Read the model definition and answer for the solid it produces. Units are mm, in the model's axes. Give positions to 0.01 mm unless a question says otherwise; leave off trailing zeros. Order: outer loops, then holes, each group sorted by start corner. A loop starts at its lowest first (then second) coordinate and runs counter-clockwise, first axis right, second up. Notation, with made-up numbers: (46.25, 41) - (77.25, 41) arc R31 ccw to (77.25, 70) - close; hole circle Ø9 at (77.5, 19). An arc over 180 degrees is marked (long way). Use a Markdown table: item, result. Add a question column.
1. A cutting plane is placed at B-B on x = 126.5. Determine the outline of the cut face in (y, z), and give its area (3 significant figures).
2. A flat-ended cylindrical pin translates along its axis: P1, Ø6, axis at x = 304.5, z = 17.5, coming from the +Y side. Find the tip coordinate at first contact, or state that the pin passes through.
3. A cutting plane is placed at A-A on z = 108.5. Determine the outline of the cut face in (x, y), and give its area (3 significant figures).
4. A cutting plane is placed at D-D on y = 2.55. State how many separate pieces and enclosed holes the cut face has, and give its area (3 significant figures).
5. Consider L1, parallel to Z at x = 110.5, y = 1; L2, parallel to X at y = 0.9, z = 93; L3, parallel to Z at x = 262, y = 2.75. Determine where each line is inside the solid, lowest interval first.
6. A cutting plane is placed at C-C on x = 291. Determine the outline of the cut face in (y, z), and give its area (3 significant figures).
```python
from build123d import *

# Parameters (mm, degrees)
SKETCH1_W           = 334.17
SKETCH1_H           = 162.4
BOSS_EXTRUDE1_DEPTH = 3
SKETCH2_R           = 5
CUT_EXTRUDE1_DEPTH  = 17
SKETCH3_W           = 3
SKETCH3_H           = 9.7
CUT_EXTRUDE3_DEPTH  = 45


with BuildPart() as part:
    # Sketch1 → Boss-Extrude1 (new body)
    with BuildSketch(Plane(origin=(0, 0, 0), x_dir=(1, 0, 0), z_dir=(0, 1, 0))):
        with Locations((167.085, -81.2)):
            Rectangle(SKETCH1_W, SKETCH1_H)
    extrude(amount=BOSS_EXTRUDE1_DEPTH)

    # Sketch2 → Cut-Extrude1 (cut)
    with BuildSketch(Plane(origin=(0, 0, 0), x_dir=(1, 0, 0), z_dir=(0, 1, 0))):
        with Locations((210, -17.5)):
            Circle(SKETCH2_R)
        with Locations((223.5, -17.5)):
            Circle(SKETCH2_R)
        with Locations((237, -17.5)):
            Circle(SKETCH2_R)
        with Locations((250.5, -17.5)):
            Circle(SKETCH2_R)
        with Locations((264, -17.5)):
            Circle(SKETCH2_R)
        with Locations((277.5, -17.5)):
            Circle(SKETCH2_R)
        with Locations((291, -17.5)):
            Circle(SKETCH2_R)
        with Locations((304.5, -17.5)):
            Circle(SKETCH2_R)
        with Locations((223.5, -35)):
            Circle(SKETCH2_R)
        with Locations((237, -35)):
            Circle(SKETCH2_R)
        with Locations((250.5, -35)):
            Circle(SKETCH2_R)
        with Locations((264, -35)):
            Circle(SKETCH2_R)
        with Locations((277.5, -35)):
            Circle(SKETCH2_R)
        with Locations((291, -35)):
            Circle(SKETCH2_R)
        with Locations((304.5, -35)):
            Circle(SKETCH2_R)
        with Locations((210, -35)):
            Circle(SKETCH2_R)
        with Locations((318, -17.5)):
            Circle(SKETCH2_R)
        with Locations((318, -35)):
            Circle(SKETCH2_R)
        with BuildLine():
            Line((210, -47.5), (255, -47.5))
            ThreePointArc((255, -47.5), (260, -52.5), (255, -57.5))
            Line((255, -57.5), (210, -57.5))
            ThreePointArc((210, -57.5), (205, -52.5), (210, -47.5))
        make_face()
        with BuildLine():
            Line((275, -57.5), (320, -57.5))
            ThreePointArc((320, -57.5), (325, -52.5), (320, -47.5))
            Line((320, -47.5), (275, -47.5))
            ThreePointArc((275, -47.5), (270, -52.5), (275, -57.5))
        make_face()
        with BuildLine():
            Line((15, -17.2), (60, -17.2))
            ThreePointArc((60, -17.2), (65, -12.2), (60, -7.2))
            Line((60, -7.2), (15, -7.2))
            ThreePointArc((15, -7.2), (10, -12.2), (15, -17.2))
        make_face()
        with BuildLine():
            Line((95, -7.2), (140, -7.2))
            ThreePointArc((140, -7.2), (145, -12.2), (140, -17.2))
            Line((140, -17.2), (95, -17.2))
            ThreePointArc((95, -17.2), (90, -12.2), (95, -7.2))
        make_face()
    cut_extrude1 = extrude(amount=CUT_EXTRUDE1_DEPTH, mode=Mode.SUBTRACT)

    # Mirror1: Cut-Extrude1 across plane
    add(cut_extrude1.mirror(Plane.XY.offset(81.2)), mode=Mode.SUBTRACT)

    # Sketch3 → Cut-Extrude3 (cut)
    with BuildSketch(Plane(origin=(0, 0, 0), x_dir=(1, 0, 0), z_dir=(0, 1, 0))):
        with Locations((204.7, -69.2)):
            Rectangle(SKETCH3_W, SKETCH3_H)
        with Locations((204.7, -93.2)):
            Rectangle(SKETCH3_W, SKETCH3_H)
    extrude(amount=CUT_EXTRUDE3_DEPTH, mode=Mode.SUBTRACT)


solid = part.part
```
Output values:
| question | item | result |
|---|---|---|
| 1 | outline | (0, 0) - (3, 0) - (3, 7.2) - (0, 7.2) - close; (0, 17.2) - (3, 17.2) - (3, 145.2) - (0, 145.2) - close; (0, 155.2) - (3, 155.2) - (3, 162.4) - (0, 162.4) - close |
| 1 | area | 427 mm² |
| 2 | P1 | through |
| 3 | outline | (0, 0) - (205.2, 0) - (205.2, 3) - (0, 3) - close; (259.8, 0) - (270.2, 0) - (270.2, 3) - (259.8, 3) - close; (324.8, 0) - (334.17, 0) - (334.17, 3) - (324.8, 3) - close |
| 3 | area | 675 mm² |
| 4 | separate pieces | 1 |
| 4 | enclosed holes | 46 |
| 4 | area | 47,200 mm² |
| 5 | L1 | 0 to 7.2, 17.2 to 145.2, 155.2 to 162.4 |
| 5 | L2 | 0 to 203.2, 206.2 to 334.17 |
| 5 | L3 | 0 to 12.92, 22.08 to 30.42, 39.58 to 122.82, 131.98 to 140.32, 149.48 to 162.4 |
| 6 | outline | (0, 0) - (3, 0) - (3, 12.5) - (0, 12.5) - close; (0, 22.5) - (3, 22.5) - (3, 30) - (0, 30) - close; (0, 40) - (3, 40) - (3, 47.5) - (0, 47.5) - close; (0, 57.5) - (3, 57.5) - (3, 104.9) - (0, 104.9) - close; (0, 114.9) - (3, 114.9) - (3, 122.4) - (0, 122.4) - close; (0, 132.4) - (3, 132.4) - (3, 139.9) - (0, 139.9) - close; (0, 149.9) - (3, 149.9) - (3, 162.4) - (0, 162.4) - close |
| 6 | area | 307 mm² |
